The model under review builds one solid part; all positions refer to its coordinate system, in mm. Face numbers are marked on the shaded views. A direction names the side the tool comes from. Coordinates: 2 decimals unless noted, no trailing zeros. Loops run counter-clockwise (first coordinate to the right, second up) from the corner with the lowest first, then second, coordinate; pieces in that order, holes last. Notation, with made-up numbers: M 53.5,59 L 76.5,59 A15 cw 76.5,64 Z; hole C -34,-38.75 d10. An arc over 180 degrees is marked long. Return JSON: item names as keys, results as strings.
```python
from build123d import *

# Parameters (mm, degrees)
F0_R     = 7.9
F1_DEPTH = 2.4
F2_R     = 1
F3_DEPTH = 4.5
F4_R     = 2
F5_SIZE  = 1


with BuildPart() as f1:
    # F0 (on Top) → F1 (new body)
    with BuildSketch(Plane.XY):
        Circle(F0_R)
    extrude(amount=-F1_DEPTH)

    # F2 (on face) → F3 (join)
    with BuildSketch(Plane.XY):
        Circle(F2_R)
    extrude(amount=F3_DEPTH)

    # F4
    f4_edges = [f1.edges().sort_by_distance(p)[0] for p in [
        (-7.9, 0, -2.4),
    ]]
    fillet(f4_edges, radius=F4_R)

    # F5
    f5_edges = [f1.edges().sort_by_distance(p)[0] for p in [
        (-1, 0, 4.5),
    ]]
    chamfer(f5_edges, length=F5_SIZE)


solid = f1.part
```
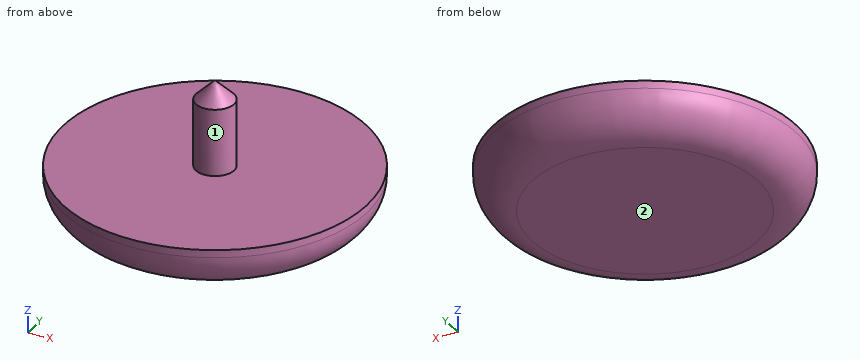
1. To check wall thickness, follow line 1 (Z direction, x = -3.5, y = 1.75); line 2 (Y direction, x = -6.5, z = -1.5); line 3 (Y direction, x = 0.25, z = 3.25). State the ranges of each line that lie inside material, in increasing order.
Check values:
{"line 1": "-2.4 to 0", "line 2": "-3.88 to 3.88", "line 3": "-0.97 to 0.97"}
2. Add section A-A on z = 3.75. Give the boundary of the cut face in (x, y), plus the area to 3 significant figures.
Check values:
{"outline": "C 0,0 d1.5", "area": "1.77 mm²"}
3. Add section B-B on z = 0.25. Give the boundary of the cut face in (x, y).
Check values:
{"outline": "C 0,0 d2"}
4. Machinability: for the marked faces 1 and 2, which of the approach directions +Z, -Z, +X, -X, +Y, -Y give a long, thin tool a straight path to every point of the face, cutting with its end or side? Answer none if there is none.
Check values:
{"face 1": "+Z", "face 2": "-Z, +X, -X, +Y, -Y"}
5. Insertion check: pin 1 Ø2 at (x, y) = (4.5, 0.5) entering from +Z; pin 2 Ø3 at (y, z) = (-3, 3) entering from -X; pin 3 Ø2 at (x, z) = (-3.5, -1) entering from -Y. Each pin has a flat end and moves straight along its axis. Give the tip position at first contact, or say it passes through.
Check values:
{"pin 1": "z = 0", "pin 2": "through", "pin 3": "y = -7.46"}
